For this review, take the finished solid that the model builds, in its own axes (mm). A direction names the side the tool comes from. Give positions to 0.01 mm unless a question says otherwise; leave off trailing zeros. Loops run counter-clockwise (first coordinate to the right, second up) from the corner with the lowest first, then second, coordinate; pieces in that order, holes last. Notation, with made-up numbers: (5, -13) -> (45, -13) arc R17 ccw to (45, 12) -> close; hole circle Ø9 at (-5, 8). An arc over 180 degrees is marked (long way). One line per question, with ' | ' between items. Start each with the question number.
(1) Insertion check: P1, Ø0.6, axis at y = 1, z = -35.5, coming from the -X side. The pin has a flat end and moves straight along its axis. Give the tip position at first contact, or say it passes through.
(2) Consider section B-B (z = 38). Write out the cut boundary in (x, y), and give its area (3 significant figures).
(3) Tool access review of faces 1 (the flat face through (11, 1, -23)), 2 (the flat face through (-23, 1, 0)), 3 (the flat face through (-3, 1, -36)), 4 (the flat face through (10, 1, 38)): name each direction out of +Z, -Z, +X, -X, +Y, -Y from which nothing blocks a thin tool from reaching the whole face with its end or side.
(4) Consider section C-C (z = -6). Write out the cut boundary in (x, y).
(5) Draft analysis for pull direction X (two halves, no side actions). For faces 5 (the cylindrical face through (4.1, 1, 36.8)), 6 (the cylindrical face through (-21.726, 1.014, 21.02)), 7 (the flat face through (23, 1, 0)), state which applies: +X half, -X half, draft (parallel to the pull), parting line (faces both ways), or undercut.
(6) Consider section A-A (x = 0). Write out the cut boundary in (y, z).
(7) Consider section D-D (z = 15.5). Write out the cut boundary in (x, y), and give its area (3 significant figures).
(8) Wall thickness on probe 1 along X at (y, z) = (1.1, 38); probe 2 along X at (y, z) = (0.5, 0); probe 3 along X at (y, z) = (0.8, -15.5): over which ranges is each line inside the solid? List them lowest first.
from build123d import *

# Parameters (mm, degrees)
SKETCH_2_W          = 46
SKETCH_2_H          = 46
SKETCH_2_R          = 18.5
EXTRUDE_1_DEPTH     = 2
FILLET_1_R          = 5.5
SKETCH_3_R          = 1.6
CUT_EXTRUDE_1_DEPTH = 33.588341474
SKETCH_4_W          = 20
SKETCH_4_H          = 20
SKETCH_4_R          = 1.5
EXTRUDE_2_DEPTH     = 2
SKETCH_5_W          = 6
SKETCH_5_H          = 27.4
SKETCH_5_R          = 1.5
EXTRUDE_3_DEPTH     = 2
FILLET_5_R          = 2
FILLET_6_R          = 10


with BuildPart() as part:
    # 草图2 → 凸台-拉伸1 (new body)
    with BuildSketch(Plane(origin=(0, 0, 0), x_dir=(1, 0, 0), z_dir=(0, 1, 0))):
        Rectangle(SKETCH_2_W, SKETCH_2_H)
        with Locations(Location((0, 0, 0), (0, 0, 270))):
            Circle(SKETCH_2_R, mode=Mode.SUBTRACT)
    extrude(amount=EXTRUDE_1_DEPTH)

    # 圆角1
    fillet_1_edges = [part.edges().sort_by_distance(p)[0] for p in [
        (23, 1, 23),
        (-23, 1, 23),
        (-23, 1, -23),
        (23, 1, -23),
    ]]
    fillet(fillet_1_edges, radius=FILLET_1_R)

    # 草图3 → 切除-拉伸1 (cut, through all)
    with BuildSketch(Plane(origin=(0, 2, 0), x_dir=(1, 0, 0), z_dir=(0, 1, 0))):
        with Locations(Location((-15.5, 15.5, 0), (0, 0, 270))):
            Circle(SKETCH_3_R)
        with Locations(Location((15.5, 15.5, 0), (0, 0, 270))):
            Circle(SKETCH_3_R)
        with Locations(Location((-15.5, -15.5, 0), (0, 0, 270))):
            Circle(SKETCH_3_R)
        with Locations(Location((15.5, -15.5, 0), (0, 0, 270))):
            Circle(SKETCH_3_R)
    extrude(amount=-CUT_EXTRUDE_1_DEPTH, mode=Mode.SUBTRACT)

    # 草图4 → 凸台-拉伸2 (add)
    with BuildSketch(Plane(origin=(0, 2, 0), x_dir=(1, 0, 0), z_dir=(0, 1, 0))):
        with Locations((0, -33)):
            Rectangle(SKETCH_4_W, SKETCH_4_H)
        with Locations(Location((-5, -38, 0), (0, 0, 270))):
            Circle(SKETCH_4_R, mode=Mode.SUBTRACT)
        with Locations(Location((5, -38, 0), (0, 0, 270))):
            Circle(SKETCH_4_R, mode=Mode.SUBTRACT)
        with Locations(Location((-5, -28, 0), (0, 0, 270))):
            Circle(SKETCH_4_R, mode=Mode.SUBTRACT)
        with Locations(Location((5, -28, 0), (0, 0, 270))):
            Circle(SKETCH_4_R, mode=Mode.SUBTRACT)
    extrude(amount=-EXTRUDE_2_DEPTH)

    # 草图5 → 凸台-拉伸3 (add)
    with BuildSketch(Plane(origin=(0, 2, 0), x_dir=(1, 0, 0), z_dir=(0, 1, 0))):
        with Locations((0, 36.350013022)):
            Rectangle(SKETCH_5_W, SKETCH_5_H)
        with Locations(Location((0, 47.050013022, 0), (0, 0, 270))):
            Circle(SKETCH_5_R, mode=Mode.SUBTRACT)
        with Locations(Location((0, 27.650013022, 0), (0, 0, 270))):
            Circle(SKETCH_5_R, mode=Mode.SUBTRACT)
    extrude(amount=-EXTRUDE_3_DEPTH)

    # 圆角5
    fillet_5_edges = [part.edges().sort_by_distance(p)[0] for p in [
        (-3, 1, -50.050013022),
        (3, 1, -50.050013022),
        (3, 1, -23),
        (-3, 1, -23),
    ]]
    fillet(fillet_5_edges, radius=FILLET_5_R)

    # 圆角6
    fillet_6_edges = [part.edges().sort_by_distance(p)[0] for p in [
        (10, 1, 23),
        (-10, 1, 23),
    ]]
    fillet(fillet_6_edges, radius=FILLET_6_R)


solid = part.part
A:
1) P1: stops at x = -3
2) outline: (-10, 0) -> (-6.5, 0) -> (-6.5, 2) -> (-10, 2) -> close; (-3.5, 0) -> (3.5, 0) -> (3.5, 2) -> (-3.5, 2) -> close; (6.5, 0) -> (10, 0) -> (10, 2) -> (6.5, 2) -> close | area: 28.0 mm^2
3) face 1: -Z, +X, +Y, -Y | face 2: +Z, -Z, -X, +Y, -Y | face 3: -Z, -X, +Y, -Y | face 4: +Z, +X, +Y, -Y
4) outline: (-23, 0) -> (-17.5, 0) -> (-17.5, 2) -> (-23, 2) -> close; (17.5, 0) -> (23, 0) -> (23, 2) -> (17.5, 2) -> close
5) face 5: undercut | face 6: -X half | face 7: +X half
6) outline: (0, -50.05) -> (2, -50.05) -> (2, -48.55) -> (0, -48.55) -> close; (0, -45.55) -> (2, -45.55) -> (2, -29.15) -> (0, -29.15) -> close; (0, -26.15) -> (2, -26.15) -> (2, -18.5) -> (0, -18.5) -> close; (0, 18.5) -> (2, 18.5) -> (2, 43) -> (0, 43) -> close
7) outline: (-23, 0) -> (-17.1, 0) -> (-17.1, 2) -> (-23, 2) -> close; (-13.9, 0) -> (-10.1, 0) -> (-10.1, 2) -> (-13.9, 2) -> close; (10.1, 0) -> (13.9, 0) -> (13.9, 2) -> (10.1, 2) -> close; (17.1, 0) -> (23, 0) -> (23, 2) -> (17.1, 2) -> close | area: 38.8 mm^2
8) probe 1: x = -10 to -6.5, -3.5 to 3.5, 6.5 to 10 | probe 2: x = -23 to -18.5, 18.5 to 23 | probe 3: x = -23 to -17.1, -13.9 to -10.1, 10.1 to 13.9, 17.1 to 23
